The listing builds one solid part. Answer for the finished solid, in the listing's coordinates (mm). A direction names the side the tool comes from. Coordinates: 2 decimals unless noted, no trailing zeros. Loops run counter-clockwise (first coordinate to the right, second up) from the corner with the lowest first, then second, coordinate; pieces in that order, holes last. Notation, with made-up numbers: M 82,35.5 L 141,35.5 A31 ccw 141,67.5 Z; hole C 74,-6 d4. An arc over 180 degrees is marked long. Answer as a JSON object with one key per item and string values. Group by question number.
1. A cutting plane is placed at A-A on z = -27. Give the vertices of the cut face in (x, y), and give its area (3 significant figures).
2. A cutting plane is placed at D-D on x = 1.2. State how many separate pieces and enclosed holes the cut face has, and give its area (3 significant figures).
3. A cutting plane is placed at B-B on y = 18.5. Give the vertices of the cut face in (x, z), and give its area (3 significant figures).
4. A cutting plane is placed at C-C on z = -4.5. Give the vertices of the cut face in (x, y), and give its area (3 significant figures).
5. Determine the mould class of faces 6 (the face through (2, -3.982, -26)), 7 (the face through (2, -57.818, 13)), 8 (the face through (0, -16, 1)) for opening direction Y: released by +Y, released by -Y, zero draft, split by the parting line, or undercut.
6. Straight lines are drawn through the part: L1, parallel to Y at x = 1.3, z = -1.5; L2, parallel to Y at x = 2.5, z = -26; L3, parallel to Y at x = 2.8, z = 31.5. For each, find the intervals that lie inside material, in ascending order.
7. For faces 1 (the face through (2, -1, -21.761)), 2 (the face through (2, -55, -6.979)), 3 (the face through (2, -55, 16.964)), 4 (the face through (2, -57.818, -11)), 5 (the face through (2, -13, 43.394)), determine the directions among +Z, -Z, +X, -X, +Y, -Y from which every point of the face is accessible in a straight line to the end or side of a thin tool.
8. Given pin 1 (3 mm diameter, centred on x = 2.5, y = -55.5, fed in from +Z); pin 2 (1.5 mm diameter, centred on x = 1.5, z = 1.5, fed in from -Y); pin 3 (1.5 mm diameter, centred on x = 3, z = 25.5, fed in from -Y), each flat-ended and moving along its own axis, determine where each tip first touches the part or whether it passes through.
from build123d import *

# Parameters (mm, degrees)
F0_R     = 1.496682
F0_W     = 5.246993
F0_H     = 8.403182
F0_R_2   = 1.502637
F0_R_3   = 7.419122
F0_R_4   = 1.50217
F0_R_5   = 1.497826
F0_R_6   = 1.495866
F0_R_7   = 7.407283
F0_R_8   = 1.495199
F1_DEPTH = 5.0038


with BuildPart() as f1:
    # F0 (on Right) → F1 (new body)
    with BuildSketch(Plane.YZ):
        with BuildLine():
            ThreePointArc((26.002148, 39.583533), (24.886225, 42.27761), (22.192148, 43.393533))
            Line((22.192148, 43.393533), (-48.969212, 43.393533))
            ThreePointArc((-48.969212, 43.393533), (-51.663225, 42.277674), (-52.779212, 39.583715))
            Line((-52.779212, 39.583715), (-52.780295, 16.96425))
            Line((-52.780295, 16.96425), (-56.547852, 16.96425))
            ThreePointArc((-56.547852, 16.96425), (-57.445878, 16.592276), (-57.817852, 15.69425))
            Line((-57.817852, 15.69425), (-57.817852, 10.11156))
            ThreePointArc((-57.817852, 10.11156), (-57.445878, 9.213534), (-56.547852, 8.84156))
            Line((-56.547852, 8.84156), (-52.783472, 8.84156))
            Line((-52.783472, 8.84156), (-52.783472, 2.413221))
            Line((-52.783472, 2.413221), (-47.806354, 2.413221))
            Line((-47.806354, 2.413221), (-47.806354, 3.672259))
            Line((-47.806354, 3.672259), (-44.797333, 3.672259))
            Line((-44.797333, 3.672259), (-44.797333, -1.80733))
            Line((-44.797333, -1.80733), (-47.806354, -1.80733))
            Line((-47.806354, -1.80733), (-47.806354, -0.579965))
            Line((-47.806354, -0.579965), (-52.783472, -0.579965))
            Line((-52.783472, -0.579965), (-52.783472, -6.978519))
            Line((-52.783472, -6.978519), (-56.547852, -6.978519))
            ThreePointArc((-56.547852, -6.978519), (-57.445878, -7.350493), (-57.817852, -8.248519))
            Line((-57.817852, -8.248519), (-57.817852, -13.858365))
            ThreePointArc((-57.817852, -13.858365), (-57.445878, -14.756391), (-56.547852, -15.128365))
            Line((-56.547852, -15.128365), (-52.823355, -15.128365))
            Line((-52.823355, -15.128365), (-52.823355, -20.055671))
            Line((-52.823355, -20.055671), (-56.547852, -20.055671))
            ThreePointArc((-56.547852, -20.055671), (-57.445878, -20.427646), (-57.817852, -21.325671))
            Line((-57.817852, -21.325671), (-57.817852, -39.156467))
            ThreePointArc((-57.817852, -39.156467), (-56.701929, -41.850544), (-54.007852, -42.966467))
            Line((-54.007852, -42.966467), (22.192148, -42.966467))
            ThreePointArc((22.192148, -42.966467), (24.886225, -41.850544), (26.002148, -39.156467))
            Line((26.002148, -39.156467), (26.002148, 39.583533))
        make_face()
        with Locations((-1.237392, -37.996951)):
            Circle(F0_R, mode=Mode.SUBTRACT)
        with Locations((-1.358906, -25.962943)):
            Rectangle(F0_W, F0_H, mode=Mode.SUBTRACT)
        with Locations((6.237176, -37.701346)):
            Circle(F0_R_2, mode=Mode.SUBTRACT)
        with Locations((14.057356, -29.971829)):
            Circle(F0_R_3, mode=Mode.SUBTRACT)
        with Locations((21.865347, -22.209868)):
            Circle(F0_R_4, mode=Mode.SUBTRACT)
        with Locations((-15.942187, 38.029493)):
            Circle(F0_R_5, mode=Mode.SUBTRACT)
        with Locations((-8.460167, 32.026364)):
            Circle(F0_R_6, mode=Mode.SUBTRACT)
        with Locations((2.551726, 32.02758)):
            Circle(F0_R_7, mode=Mode.SUBTRACT)
        with Locations((13.543643, 32.025907)):
            Circle(F0_R_8, mode=Mode.SUBTRACT)
    extrude(amount=F1_DEPTH)


solid = f1.part
From the geometry:
{
 "1": {"outline": "M 0,-57.82 L 5,-57.82 L 5,-3.98 L 0,-3.98 Z; M 0,1.26 L 5,1.26 L 5,7.26 L 0,7.26 Z; M 0,20.86 L 5,20.86 L 5,26 L 0,26 Z", "area": "325 mm²"},
 "2": {"separate pieces": "1", "enclosed holes": "9", "area": "6,520 mm²"},
 "3": {"outline": "M 0,-42.97 L 5,-42.97 L 5,-35.91 L 0,-35.91 Z; M 0,-24.03 L 5,-24.03 L 5,43.39 L 0,43.39 Z", "area": "373 mm²"},
 "4": {"outline": "M 0,-52.78 L 5,-52.78 L 5,26 L 0,26 Z", "area": "394 mm²"},
 "5": {"face 6": "undercut", "face 7": "released by -Y", "face 8": "zero draft"},
 "6": {"L1": "y = -52.78 to -47.81, -44.8 to 26", "L2": "y = -57.82 to -3.98, 1.26 to 7.79, 20.32 to 26", "L3": "y = -52.78 to -9.86, -7.06 to -4.84, 9.94 to 12.14, 14.94 to 26"},
 "7": {"face 1": "+X, -X", "face 2": "+X, -X, -Y", "face 3": "+Z, +X, -X, -Y", "face 4": "+Z, -Z, +X, -X, -Y", "face 5": "+Z, +X, -X, +Y, -Y"},
 "8": {"pin 1": "stops at z = 16.96", "pin 2": "stops at y = -44.8", "pin 3": "stops at y = -52.78"}
}
